from build123d import *

# Parameters (mm, degrees)
SKETCH1_R           = 38.1
BOSS_EXTRUDE1_DEPTH = 25.4
SHELL1_T            = -2.54
FILLET1_R           = 2.54
SKETCH2_R           = 3.175
CUT_EXTRUDE1_DEPTH  = 60.568280214
CIRPATTERN1_COUNT   = 4
SKETCH3_W           = 40.812489524
SKETCH3_H           = 30.878008928
BOSS_EXTRUDE2_DEPTH = 12.7
SKETCH6_R           = 3.175
BOSS_EXTRUDE4_DEPTH = 2.54
FILLET3_R           = 7.62
SKETCH8_W           = 40.812489524
SKETCH8_H           = 1.27
BOSS_EXTRUDE7_DEPTH = 2.54
SKETCH9_W           = 15.412489524
SKETCH9_H           = 30.878008928
CUT_EXTRUDE2_DEPTH  = 2.54


with BuildPart() as part:
    # Sketch1 → Boss-Extrude1 (new body)
    with BuildSketch(Plane.XY):
        with Locations(Location((0, 0, 0), (0, 0, 180))):
            Circle(SKETCH1_R)
    extrude(amount=BOSS_EXTRUDE1_DEPTH)

    # Shell1
    shell1_openings = [part.faces().sort_by_distance(p)[0] for p in [
        (0, 0, 0),
    ]]
    offset(amount=SHELL1_T, openings=shell1_openings, kind=Kind.INTERSECTION)

    # Fillet1
    fillet1_edges = [part.edges().sort_by_distance(p)[0] for p in [
        (38.1, 0, 25.4),
    ]]
    fillet(fillet1_edges, radius=FILLET1_R)

    # Sketch2 → Cut-Extrude1 (cut, through all)
    with BuildSketch(Plane.XY.offset(25.4)):
        with Locations((0, 25.4)):
            Circle(SKETCH2_R)
    cut_extrude1 = extrude(amount=-CUT_EXTRUDE1_DEPTH, mode=Mode.SUBTRACT)

    # CirPattern1: Cut-Extrude1 ×4 about axis
    cirpattern1_axis = Axis((0, 0, 0), (0, 0, 1))
    for i in range(1, CIRPATTERN1_COUNT):
        add(cut_extrude1.rotate(cirpattern1_axis, i * 360 / CIRPATTERN1_COUNT), mode=Mode.SUBTRACT)

    # Sketch3 → Boss-Extrude2 (add)
    with BuildSketch(Plane.XY.offset(25.4)):
        Rectangle(SKETCH3_W, SKETCH3_H)
    extrude(amount=BOSS_EXTRUDE2_DEPTH)

    # Sketch6 → Boss-Extrude4 (add)
    with BuildSketch(Plane.XY.offset(25.4)):
        with Locations((25.4, 0)):
            Circle(SKETCH6_R)
        with Locations((-25.4, 0)):
            Circle(SKETCH6_R)
    extrude(amount=-BOSS_EXTRUDE4_DEPTH)

    # Fillet3
    fillet3_edges = [part.edges().sort_by_distance(p)[0] for p in [
        (20.406244762, 0, 25.4),
        (-20.406244762, 0, 25.4),
    ]]
    fillet(fillet3_edges, radius=FILLET3_R)

    # Sketch8 → Boss-Extrude7 (add)
    with BuildSketch(Plane.XY.offset(38.1)):
        with Locations((0, 14.804004464)):
            Rectangle(SKETCH8_W, SKETCH8_H)
        with Locations((0, 9.724004464)):
            Rectangle(SKETCH8_W, SKETCH8_H)
        with Locations((0, -9.724004464)):
            Rectangle(SKETCH8_W, SKETCH8_H)
        with Locations((0, -14.804004464)):
            Rectangle(SKETCH8_W, SKETCH8_H)
    extrude(amount=BOSS_EXTRUDE7_DEPTH)

    # Sketch9 → Cut-Extrude2 (cut)
    with BuildSketch(Plane.XY.offset(40.64)):
        Rectangle(SKETCH9_W, SKETCH9_H)
    extrude(amount=-CUT_EXTRUDE2_DEPTH, mode=Mode.SUBTRACT)


solid = part.part
The listing builds one solid part. Answer for the finished solid, in the listing's coordinates (mm). A direction names the side the tool comes from. Round coordinates to 2 decimals unless told otherwise and drop trailing zeros. Write each loop counter-clockwise with the first axis right and the second up, starting at its lowest first coordinate (ties: lowest second). Pieces come first, ordered by that corner, then holes. Notation, with made-up numbers: M 27,-19.5 L 54,-19.5 A35 cw 54,13.5 Z; hole C 5,69.5 d4. An arc over 180 degrees is marked long. Write each question's results on one line, items separated by ' | '. Start each with the question number.
(1) The part is cut by section D-D, the plane z = 32. Write down the section's boundary in (x, y).
(2) For faces 1 (the flat face through (0, -15.439, 33)), 2 (the flat face through (14, 10.359, 39)), 3 (the flat face through (-20.406, 0, 36)), determine the directions among +Z, -Z, +X, -X, +Y, -Y from which every point of the face is accessible in a straight line to the end or side of a thin tool.
(3) The part is cut by section B-B, the plane y = 0. Write down the section's boundary in (x, z), and give its area (3 significant figures).
(4) Find the intervals of material crossed by line 1 (Y direction, x = 0, z = 23) (3 decimals); line 2 (Y direction, x = 0, z = 24.55) (3 decimals); line 3 (Z direction, x = -16, y = -1), in increasing order.
(5) The part is cut by section C-C, the plane z = 10.5. Write down the section's boundary in (x, y).
(6) Determine the mould class of faces 4 (the cylindrical face through (-22.7, 0.22, 27.57)), 5 (the flat face through (0, 15.439, 33)), 6 (the cylindrical face through (0.41, -28.55, 24.15)) for opening direction Y: +Y half, -Y half, draft (parallel to the pull), parting line (faces both ways), or undercut.
(7) Each of these flat-tipped pins is pushed along its axis until it touches: P1, Ø5, axis at y = -18.5, z = 22.5, coming from the -X side; P2, Ø2, axis at x = -13, z = 30.5, coming from the -Y side; P3, Ø3, axis at x = 0, z = 31.5, coming from the +Y side; P4, Ø5.5, axis at x = 0, y = -25.4, coming from the -Z side. Where does it stop, or does it pass through?
(8) The part is cut by section A-A, the plane x = 0. Write down the section's boundary in (y, z) (3 decimals).
Worked answers:
1) outline: M -20.47,-15.44 L 20.47,-15.44 L 20.47,15.44 L -20.47,15.44 Z
2) face 1: +Z, +X, -X, -Y | face 2: +Z, +X, -X | face 3: +Z, -X, +Y, -Y
3) outline: M -38.1,0 L -35.56,0 L -35.56,22.86 L 35.56,22.86 L 35.56,0 L 38.1,0 L 38.1,22.86 A2.54 ccw 35.56,25.4 L 28.03,25.4 A7.62 cw 20.41,33.02 L 20.41,38.1 L -20.41,38.1 L -20.41,33.02 A7.62 cw -28.03,25.4 L -35.56,25.4 A2.54 ccw -38.1,22.86 Z | area: 850 mm²
4) line 1: y = -38.096 to -28.575, -22.225 to 22.225, 28.575 to 38.096 | line 2: y = -37.456 to -28.575, -22.225 to 22.225, 28.575 to 37.456 | line 3: z = 22.86 to 38.1
5) outline: C 0,0 d76.2; hole C 0,0 d71.12
6) face 4: draft | face 5: +Y half | face 6: undercut
7) P1: stops at x = -34.58 | P2: stops at y = -15.44 | P3: stops at y = 15.44 | P4: passes through
8) outline: M -38.1,0 L -35.56,0 L -35.56,22.86 L -28.575,22.86 L -28.575,25.4 L -35.56,25.4 A2.54 ccw -38.1,22.86 Z; M -22.225,22.86 L 22.225,22.86 L 22.225,25.4 L 15.439,25.4 L 15.439,38.1 L -15.439,38.1 L -15.439,25.4 L -22.225,25.4 Z; M 28.575,22.86 L 35.56,22.86 L 35.56,0 L 38.1,0 L 38.1,22.86 A2.54 ccw 35.56,25.4 L 28.575,25.4 Z
